from build123d import *

# Parameters (mm, degrees)
F1_DEPTH = 5
F2_R     = 16.0925
F3_DEPTH = 5


with BuildPart() as f1:
    # F0 (on Top) → F1 (new body)
    with BuildSketch(Plane.XY):
        with BuildLine():
            ThreePointArc((19.224025974, -0.9996626181), (19.2435053979, -0.5), (19.25, 0))
            ThreePointArc((19.25, 0), (19.2435053979, 0.5), (19.224025974, 0.9996626181))
            ThreePointArc((19.224025974, 0.9996626181), (18.25, 0), (19.224025974, -0.9996626181))
        make_face()
        with BuildLine():
            ThreePointArc((19.224025974, 0.9996626181), (19.2435053979, 0.5), (19.25, 0))
            ThreePointArc((19.25, 0), (19.2435053979, -0.5), (19.224025974, -0.9996626181))
            ThreePointArc((19.224025974, -0.9996626181), (19.9478631578, -0.716231117), (20.25, 0))
            ThreePointArc((20.25, 0), (19.9478631578, 0.716231117), (19.224025974, 0.9996626181))
        make_face()
        with BuildLine():
            ThreePointArc((19.224025974, -0.9996626181), (18.25, 0), (19.224025974, 0.9996626181))
            ThreePointArc((19.224025974, 0.9996626181), (17.7038739711, 7.558792656), (14.0179049045, 13.1932119702))
            ThreePointArc((14.0179049045, 13.1932119702), (12.6222310158, 13.1811146792), (12.5738865363, 14.5760034774))
            ThreePointArc((12.5738865363, 14.5760034774), (7.1736557935, 17.8634028829), (0.9996626181, 19.224025974))
            ThreePointArc((0.9996626181, 19.224025974), (0, 18.25), (-0.9996626181, 19.224025974))
            ThreePointArc((-0.9996626181, 19.224025974), (-7.4690346519, 17.7419283442), (-13.0505499689, 14.1508178388))
            ThreePointArc((-13.0505499689, 14.1508178388), (-12.8411799857, 13.8300006906), (-12.7678002695, 13.4540022202))
            ThreePointArc((-12.7678002695, 13.4540022202), (-13.3678605948, 12.5374607554), (-14.4478967828, 12.7208796298))
            ThreePointArc((-14.4478967828, 12.7208796298), (-17.8268428947, 7.2640327922), (-19.224025974, 0.9996626181))
            ThreePointArc((-19.224025974, 0.9996626181), (-18.533768883, 0.6978631578), (-18.25, 0))
            ThreePointArc((-18.25, 0), (-18.533768883, -0.6978631578), (-19.224025974, -0.9996626181))
            ThreePointArc((-19.224025974, -0.9996626181), (-17.7419283442, -7.4690346519), (-14.1508178388, -13.0505499689))
            ThreePointArc((-14.1508178388, -13.0505499689), (-13.0646538021, -12.8467097151), (-12.4540022202, -13.7678002695))
            ThreePointArc((-12.4540022202, -13.7678002695), (-12.5231094792, -14.1330928984), (-12.7208796298, -14.4478967828))
            ThreePointArc((-12.7208796298, -14.4478967828), (-7.2640327922, -17.8268428947), (-0.9996626181, -19.224025974))
            ThreePointArc((-0.9996626181, -19.224025974), (0, -18.25), (0.9996626181, -19.224025974))
            ThreePointArc((0.9996626181, -19.224025974), (7.558792656, -17.7038739711), (13.1932119702, -14.0179049045))
            ThreePointArc((13.1932119702, -14.0179049045), (13.1811146792, -12.6222310158), (14.5760034774, -12.5738865363))
            ThreePointArc((14.5760034774, -12.5738865363), (17.8634028829, -7.1736557935), (19.224025974, -0.9996626181))
        make_face()
        with BuildLine():
            ThreePointArc((12.5738865363, 14.5760034774), (12.6222310158, 13.1811146792), (14.0179049045, 13.1932119702))
            ThreePointArc((14.0179049045, 13.1932119702), (13.3138601125, 13.9033675383), (12.5738865363, 14.5760034774))
        make_face()
        with BuildLine():
            ThreePointArc((12.5738865363, 14.5760034774), (13.3138601125, 13.9033675383), (14.0179049045, 13.1932119702))
            ThreePointArc((14.0179049045, 13.1932119702), (14.2369107048, 13.5186889659), (14.3138601125, 13.9033675383))
            ThreePointArc((14.3138601125, 13.9033675383), (13.6744335612, 14.8360983612), (12.5738865363, 14.5760034774))
        make_face()
        with BuildLine():
            ThreePointArc((14.9033675383, -13.3138601125), (14.8178717589, -12.9092837533), (14.5760034774, -12.5738865363))
            ThreePointArc((14.5760034774, -12.5738865363), (13.9033675383, -13.3138601125), (13.1932119702, -14.0179049045))
            ThreePointArc((13.1932119702, -14.0179049045), (14.2840540444, -14.2385642728), (14.9033675383, -13.3138601125))
        make_face()
        with BuildLine():
            ThreePointArc((13.1932119702, -14.0179049045), (13.9033675383, -13.3138601125), (14.5760034774, -12.5738865363))
            ThreePointArc((14.5760034774, -12.5738865363), (13.1811146792, -12.6222310158), (13.1932119702, -14.0179049045))
        make_face()
        with BuildLine():
            ThreePointArc((-0.9996626181, 19.224025974), (0, 18.25), (0.9996626181, 19.224025974))
            ThreePointArc((0.9996626181, 19.224025974), (0, 19.25), (-0.9996626181, 19.224025974))
        make_face()
        with BuildLine():
            ThreePointArc((-0.9996626181, 19.224025974), (0, 19.25), (0.9996626181, 19.224025974))
            ThreePointArc((0.9996626181, 19.224025974), (0.999915651, 19.2370118915), (1, 19.25))
            ThreePointArc((1, 19.25), (-0.0129881085, 20.249915651), (-0.9996626181, 19.224025974))
        make_face()
        with BuildLine():
            ThreePointArc((1, -19.25), (0.999915651, -19.2370118915), (0.9996626181, -19.224025974))
            ThreePointArc((0.9996626181, -19.224025974), (0, -19.25), (-0.9996626181, -19.224025974))
            ThreePointArc((-0.9996626181, -19.224025974), (-0.0129881085, -20.249915651), (1, -19.25))
        make_face()
        with BuildLine():
            ThreePointArc((-0.9996626181, -19.224025974), (0, -19.25), (0.9996626181, -19.224025974))
            ThreePointArc((0.9996626181, -19.224025974), (0, -18.25), (-0.9996626181, -19.224025974))
        make_face()
        with BuildLine():
            ThreePointArc((-12.7678002695, 13.4540022202), (-12.8411799857, 13.8300006906), (-13.0505499689, 14.1508178388))
            ThreePointArc((-13.0505499689, 14.1508178388), (-13.7678002695, 13.4540022202), (-14.4478967828, 12.7208796298))
            ThreePointArc((-14.4478967828, 12.7208796298), (-13.3678605948, 12.5374607554), (-12.7678002695, 13.4540022202))
        make_face()
        with BuildLine():
            ThreePointArc((-14.4478967828, 12.7208796298), (-13.7678002695, 13.4540022202), (-13.0505499689, 14.1508178388))
            ThreePointArc((-13.0505499689, 14.1508178388), (-14.4830106731, 14.1529114264), (-14.4478967828, 12.7208796298))
        make_face()
        with BuildLine():
            ThreePointArc((-14.1508178388, -13.0505499689), (-14.1529114264, -14.4830106731), (-12.7208796298, -14.4478967828))
            ThreePointArc((-12.7208796298, -14.4478967828), (-13.4540022202, -13.7678002695), (-14.1508178388, -13.0505499689))
        make_face()
        with BuildLine():
            ThreePointArc((-14.1508178388, -13.0505499689), (-13.4540022202, -13.7678002695), (-12.7208796298, -14.4478967828))
            ThreePointArc((-12.7208796298, -14.4478967828), (-12.5231094792, -14.1330928984), (-12.4540022202, -13.7678002695))
            ThreePointArc((-12.4540022202, -13.7678002695), (-13.0646538021, -12.8467097151), (-14.1508178388, -13.0505499689))
        make_face()
        with BuildLine():
            ThreePointArc((-18.25, 0), (-18.533768883, 0.6978631578), (-19.224025974, 0.9996626181))
            ThreePointArc((-19.224025974, 0.9996626181), (-19.25, 0), (-19.224025974, -0.9996626181))
            ThreePointArc((-19.224025974, -0.9996626181), (-18.533768883, -0.6978631578), (-18.25, 0))
        make_face()
        with BuildLine():
            ThreePointArc((-19.224025974, -0.9996626181), (-19.25, 0), (-19.224025974, 0.9996626181))
            ThreePointArc((-19.224025974, 0.9996626181), (-20.25, 0), (-19.224025974, -0.9996626181))
        make_face()
    extrude(amount=F1_DEPTH)

    # F2 (on face) → F3 (join)
    with BuildSketch(Plane.XY.offset(5)):
        Circle(F2_R)
    extrude(amount=F3_DEPTH)


solid = f1.part
The listing builds one solid part. Answer for the finished solid, in the listing's coordinates (mm). A direction names the side the tool comes from. Give positions to 0.01 mm unless a question says otherwise; leave off trailing zeros. Write each loop counter-clockwise with the first axis right and the second up, starting at its lowest first coordinate (ties: lowest second). Pieces come first, ordered by that corner, then holes.
1) Find the intervals of material crossed by L1, parallel to Z at x = 12.5, y = -11; L2, parallel to X at y = 5, z = 6.5; L3, parallel to Y at x = -4.5, z = 9.25, in increasing order.
2) For a pull along X with two mould halves and no side action, classify faces 1 (the face through (-14.169, -14.467, 2.465)), 2 (the face through (17.74, 7.47, 2.46)), 3 (the face through (-14.467, 14.169, 2.465)), 4 (the face through (0, 0, 10)) as pulls with the +X half, pulls with the -X half, needs draft (parallel to the pull), parting line crosses it, or undercut.
3) A tool of negligible diameter and unlimited length cuts with its end or side. For faces 5 (the face through (0, 0, 0)), 6 (the face through (-14, -9, 5)), from which of +Z, -Z, +X, -X, +Y, -Y can it reach the whole face along a straight path? Write none if from no direction.
4) Section B-B (x = -7) is taken. Write down the section's boundary in (y, z).
5) Given P1, Ø6, axis at x = -9.5, z = 3.5, coming from the +Y side; P2, Ø4, axis at x = 13.5, z = 3.5, coming from the +Y side; P3, Ø1.5, axis at y = -9, z = 7.5, coming from the -X side, each flat-ended and moving along its own axis, determine where each tip first touches the part or whether it passes through.
6) Section A-A (z = 0.75) is taken. Write down the section's boundary in (x, y), and give its area (3 significant figures).
7) Section C-C (y = 9.5) is taken. Write down the section's boundary in (x, z), and give its area (3 significant figures).
8) Section D-D (z = 9.25) is taken. Write down the section's boundary in (x, y) (1 decimal), and give its area (3 significant figures).
Response:
1. L1: z = 0 to 5
1. L2: x = -15.3 to 15.3
1. L3: y = -15.45 to 15.45
2. face 1: undercut
2. face 2: pulls with the +X half
2. face 3: undercut
2. face 4: needs draft
3. face 5: -Z, +X, -X, +Y, -Y
3. face 6: +Z
4. outline: (-17.93, 0) - (17.93, 0) - (17.93, 5) - (14.49, 5) - (14.49, 10) - (-14.49, 10) - (-14.49, 5) - (-17.93, 5) - close
5. P1: stops at y = 18.12
5. P2: stops at y = 15.44
5. P3: stops at x = -13.82
6. outline: (-19.22, -1) arc R19.25 ccw to (-14.15, -13.05) arc R1 ccw (long way) to (-12.72, -14.45) arc R19.25 ccw to (-1, -19.22) arc R1 ccw (long way) to (1, -19.22) arc R19.25 ccw to (13.19, -14.02) arc R1 ccw (long way) to (14.58, -12.57) arc R19.25 ccw to (19.22, -1) arc R1 ccw (long way) to (19.22, 1) arc R19.25 ccw to (14.02, 13.19) arc R1 ccw (long way) to (12.57, 14.58) arc R19.25 ccw to (1, 19.22) arc R1 ccw (long way) to (-1, 19.22) arc R19.25 ccw to (-13.05, 14.15) arc R1 ccw (long way) to (-14.45, 12.72) arc R19.25 ccw to (-19.22, 1) arc R1 ccw (long way) to start
6. area: 1,180 mm2
7. outline: (-16.74, 0) - (16.74, 0) - (16.74, 5) - (12.99, 5) - (12.99, 10) - (-12.99, 10) - (-12.99, 5) - (-16.74, 5) - close
7. area: 297 mm2
8. outline: circle Ø32.2 at (0, 0)
8. area: 814 mm2
